```python
from build123d import *

# Parameters (mm, degrees)
F0_W     = 203.2
F0_H     = 254
F0_W_2   = 190.5
F0_H_2   = 241.3
F1_DEPTH = 152.4
F2_W     = 203.2
F2_H     = 254
F3_DEPTH = 6.35
F4_R     = 6.35
F5_W     = 63.5
F5_H     = 38.1
F5_R     = 4.7625
F6_DEPTH = 12.7


with BuildPart() as f1:
    # F0 (on Front) → F1 (new body)
    with BuildSketch(Plane.XZ):
        Rectangle(F0_W, F0_H)
        Rectangle(F0_W_2, F0_H_2, mode=Mode.SUBTRACT)
    extrude(amount=F1_DEPTH)

    # F2 (on face) → F3 (join)
    with BuildSketch(Plane(origin=(0, 0, 0), x_dir=(-1, 0, 0), z_dir=(0, 1, 0))):
        Rectangle(F2_W, F2_H)
    extrude(amount=F3_DEPTH)

    # F4
    f4_edges = [f1.edges().sort_by_distance(p)[0] for p in [
        (-95.25, 0, 0),
        (95.25, 0, 0),
        (-101.6, 6.35, 0),
        (101.6, 6.35, 0),
    ]]
    fillet(f4_edges, radius=F4_R)

    # F5 (on face) → F6 (join)
    with BuildSketch(Plane.XZ.offset(152.4)):
        with Locations((0, 139.7)):
            Rectangle(F5_W, F5_H)
        with Locations((-14.2875, 144.4625)):
            Circle(F5_R, mode=Mode.SUBTRACT)
        with Locations((14.2875, 144.4625)):
            Circle(F5_R, mode=Mode.SUBTRACT)
    extrude(amount=-F6_DEPTH)


solid = f1.part
```
Verification items for the finished model (mm, model axes). A direction names the side the tool comes from. Coordinates: 2 decimals unless noted, no trailing zeros. Order: outer loops, then holes, each group sorted by start corner. A loop starts at its lowest first (then second) coordinate and runs counter-clockwise, first axis right, second up. Notation, with made-up numbers: (43.5, -15) - (88.5, -15) arc R35 ccw to (88.5, 18) - close; hole circle Ø8 at (73, 22). An arc over 180 degrees is marked (long way). Return JSON: item names as keys, results as strings.
(1) Thickness scan on line 1 along Z through (x, y) = (-66.5, -72); line 2 along X through (y, z) = (-125, 14); line 3 along Y through (x, z) = (17, 81). Record the ranges inside material, lowest first.
Filled sheet:
{"line 1": "z = -127 to -120.65, 120.65 to 127", "line 2": "x = -101.6 to -95.25, 95.25 to 101.6", "line 3": "y = 0 to 6.35"}
(2) Mould release check, pull along X, two halves, no side actions. Record for faces 1 (the flat face through (95.25, -78, -2)), 2 (the flat face through (1, -74, 127)), 3 (the cylindrical face through (99.79, 4.44, 1.78)): pulls with the +X half, pulls with the -X half, needs draft (parallel to the pull), parting line crosses it, or undercut.
Filled sheet:
{"face 1": "undercut", "face 2": "needs draft", "face 3": "pulls with the +X half"}
(3) Go/stop test with flat-tipped pins: pin 1 (6.5 mm diameter, centred on y = -147.5, z = 147.5, fed in from -X); pin 2 (5 mm diameter, centred on x = 27, y = -134.5, fed in from +Z); pin 3 (12 mm diameter, centred on x = 78, z = -75, fed in from -Y); pin 4 (11 mm diameter, centred on x = -14.29, z = 144.46, fed in from -Y). Record where each tip stops, or that it passes through.
Filled sheet:
{"pin 1": "stops at x = -31.75", "pin 2": "stops at z = 127", "pin 3": "stops at y = 0", "pin 4": "stops at y = -152.4"}
(4) Access from +Z, -Z, +X, -X, +Y, -Y to the whole of each face (thin tool, end or side, straight path). Record for faces 4 (the flat face through (-1, -75, -120.65)), 5 (the flat face through (0, -139.7, 143)), 6 (the flat face through (1, 6.35, 2)), 7 (the cylindrical face through (13.255, -146.139, 139.813)), 8 (the flat face through (-31.75, -146, 143)).
Filled sheet:
{"face 4": "-Y", "face 5": "+Z, +X, -X, +Y", "face 6": "+Z, -Z, +X, -X, +Y", "face 7": "+Y, -Y", "face 8": "+Z, -X, +Y, -Y"}
(5) Section check B-B, the plane y = -132. Record the cut outline in (x, z), and give its area (3 significant figures).
Filled sheet:
{"outline": "(-101.6, -127) - (101.6, -127) - (101.6, 127) - (-101.6, 127) - close; hole (-95.25, -120.65) - (95.25, -120.65) - (95.25, 120.65) - (-95.25, 120.65) - close", "area": "5,650 mm^2"}
(6) Section check A-A, the plane x = -83. Record the cut outline in (y, z), and give its area (3 significant figures).
Filled sheet:
{"outline": "(-152.4, -127) - (6.35, -127) - (6.35, 127) - (-152.4, 127) - (-152.4, 120.65) - (0, 120.65) - (0, -120.65) - (-152.4, -120.65) - close", "area": "3,550 mm^2"}
(7) Section check C-C, the plane z = 92. Record the cut outline in (x, y), and give its area (3 significant figures).
Filled sheet:
{"outline": "(-101.6, -152.4) - (-95.25, -152.4) - (-95.25, -6.35) arc R6.35 cw to (-88.9, 0) - (88.9, 0) arc R6.35 cw to (95.25, -6.35) - (95.25, -152.4) - (101.6, -152.4) - (101.6, 0) arc R6.35 ccw to (95.25, 6.35) - (-95.25, 6.35) arc R6.35 ccw to (-101.6, 0) - close", "area": "3,230 mm^2"}
